For this review, take the finished solid that the model builds, in its own axes (mm). Face numbers are marked on the shaded views. Round coordinates to 2 decimals unless told otherwise and drop trailing zeros. Order: outer loops, then holes, each group sorted by start corner. A loop starts at its lowest first (then second) coordinate and runs counter-clockwise, first axis right, second up. Notation, with made-up numbers: (24.25, 59.5) - (81.25, 59.5) arc R19 ccw to (81.25, 63.5) - close; hole circle Ø6 at (84.25, 20). An arc over 180 degrees is marked (long way). Write each question's results on one line, items separated by ' | '. Start each with the question number.
(1) Take a section at C-C, the plane y = 3.45. Give the boundary of the cut face in (x, z), plus the area to 3 significant figures.
(2) Take a section at A-A, the plane x = -17. Give the boundary of the cut face in (y, z).
(3) Take a section at B-B, the plane z = 0. Give the boundary of the cut face in (x, y), plus the area to 3 significant figures.
(4) Draft analysis for pull direction Z (two halves, no side actions). For the marked faces 1, 2 and 3, state which applies: pulls with the +Z half, pulls with the -Z half, needs draft (parallel to the pull), parting line crosses it, or undercut.
(5) Insertion check: pin 1 Ø4 at (x, z) = (0, 0) entering from +Y; pin 2 Ø8.5 at (x, z) = (17, 0) entering from +Y. Each pin has a flat end and moves straight along its axis. Give the tip position at first contact, or say it passes through.
(6) For L1, parallel to X at y = 1.5, z = 0; L2, parallel to X at y = 3.3, z = 3; L3, parallel to Z at x = 0.5, y = 2.7, list the stretches that pass through material, from the lowest coordinate up. Write a range as from..to.
(7) Take a section at D-D, the plane x = 0. Give the boundary of the cut face in (y, z).
```python
from build123d import *

# Parameters (mm, degrees)
SKETCH1_W           = 55
SKETCH1_H           = 25
BOSS_EXTRUDE1_DEPTH = 6
SKETCH2_R           = 3.5
SKETCH2_R_2         = 3.75
SKETCH2_R_3         = 3.95
CUT_EXTRUDE1_DEPTH  = 6
FILLET1_R           = 3.5


with BuildPart() as part:
    # Sketch1 → Boss-Extrude1 (new body)
    with BuildSketch(Plane(origin=(0, 0, 0), x_dir=(1, 0, 0), z_dir=(0, 1, 0))):
        Rectangle(SKETCH1_W, SKETCH1_H)
    extrude(amount=BOSS_EXTRUDE1_DEPTH)

    # Sketch2 → Cut-Extrude1 (cut)
    with BuildSketch(Plane(origin=(0, 6, 0), x_dir=(1, 0, 0), z_dir=(0, 1, 0))):
        with Locations(Location((0, 0, 0), (0, 0, 270))):
            Circle(SKETCH2_R)
        with Locations(Location((17, 0, 0), (0, 0, 270))):
            Circle(SKETCH2_R_2)
        with Locations(Location((-17, 0, 0), (0, 0, 270))):
            Circle(SKETCH2_R_3)
    extrude(amount=-CUT_EXTRUDE1_DEPTH, mode=Mode.SUBTRACT)

    # Fillet1
    fillet1_edges = [part.edges().sort_by_distance(p)[0] for p in [
        (27.5, 3, 12.5),
        (-27.5, 3, 12.5),
        (-27.5, 3, -12.5),
        (27.5, 3, -12.5),
    ]]
    fillet(fillet1_edges, radius=FILLET1_R)


solid = part.part
```
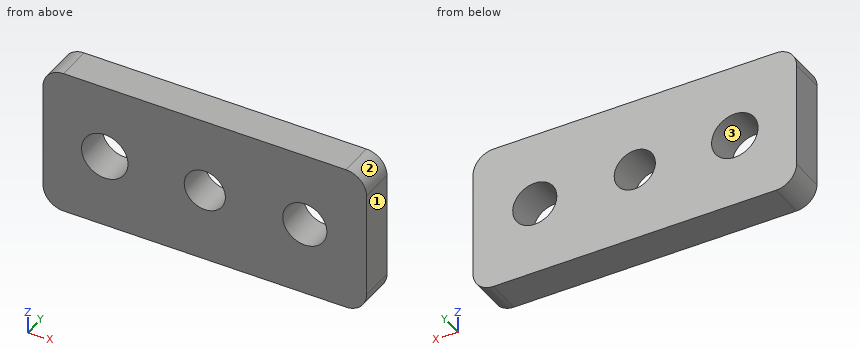
Results below:
1) outline: (-27.5, -9) arc R3.5 ccw to (-24, -12.5) - (24, -12.5) arc R3.5 ccw to (27.5, -9) - (27.5, 9) arc R3.5 ccw to (24, 12.5) - (-24, 12.5) arc R3.5 ccw to (-27.5, 9) - close; hole circle Ø7.9 at (-17, 0); hole circle Ø7 at (0, 0); hole circle Ø7.5 at (17, 0) | area: 1,230 mm^2
2) outline: (0, -12.5) - (6, -12.5) - (6, -3.95) - (0, -3.95) - close; (0, 3.95) - (6, 3.95) - (6, 12.5) - (0, 12.5) - close
3) outline: (-27.5, 0) - (-20.95, 0) - (-20.95, 6) - (-27.5, 6) - close; (-13.05, 0) - (-3.5, 0) - (-3.5, 6) - (-13.05, 6) - close; (3.5, 0) - (13.25, 0) - (13.25, 6) - (3.5, 6) - close; (20.75, 0) - (27.5, 0) - (27.5, 6) - (20.75, 6) - close | area: 196 mm^2
4) face 1: needs draft | face 2: pulls with the +Z half | face 3: undercut
5) pin 1: passes through | pin 2: stops at y = 6
6) L1: x = -27.5..-20.95, -13.05..-3.5, 3.5..13.25, 20.75..27.5 | L2: x = -27.5..-19.57, -14.43..-1.8, 1.8..14.75, 19.25..27.5 | L3: z = -12.5..-3.46, 3.46..12.5
7) outline: (0, -12.5) - (6, -12.5) - (6, -3.5) - (0, -3.5) - close; (0, 3.5) - (6, 3.5) - (6, 12.5) - (0, 12.5) - close
